Here's the drawing with two shaded views (mm, measured from the low corner). I have some questions. A direction names the side the tool comes from. Give positions to 0.01 mm unless a question says otherwise; leave off trailing zeros. Write each loop counter-clockwise with the first axis right and the second up, starting at its lowest first coordinate (ties: lowest second). Pieces come first, ordered by that corner, then holes. Notation, with made-up numbers: (15, -11.75) - (74, -11.75) arc R21 ccw to (74, 11.25) - close; hole circle Ø9 at (37, -39.5). An arc over 180 degrees is marked (long way). Answer as a JSON object with one key per item and string values. Group by question number.
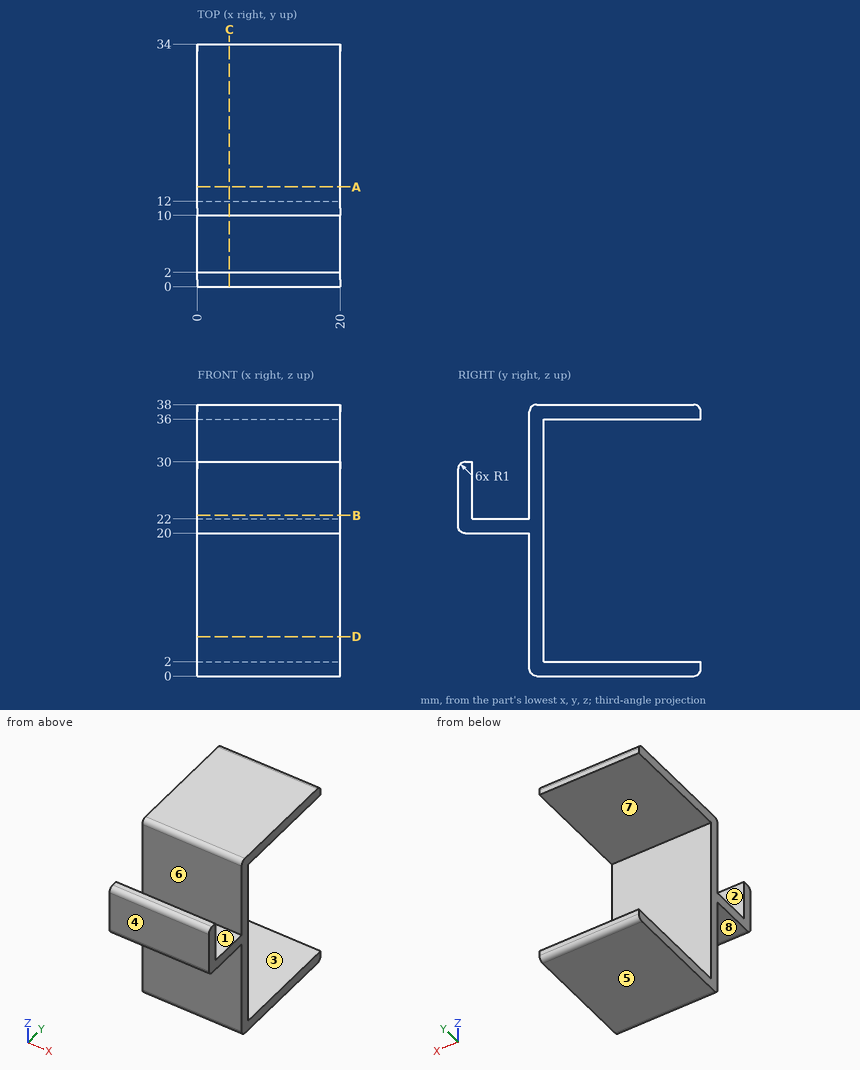
(1) I want a section at D-D, the plane z = 5.5. Please give me the cut outline in (x, y), and give its area (3 significant figures).
(2) I need wall thicknesses on L1, parallel to Z at x = 5, y = 25; L2, parallel to Y at x = 14.25, z = 3; L3, parallel to Y at x = 3.75, z = 27. Which ranges of each line are inside material? Lowest first, please.
(3) Will these pins go through, and if not, where does the flat tip stop? P1, Ø2, axis at x = 14.5, z = 15.5, coming from the -Y side; P2, Ø4, axis at x = 4, z = 29, coming from the +Y side; P3, Ø0.8, axis at x = 10.5, y = 1.5, coming from the +Z side.
(4) I want a section at B-B, the plane z = 22.5. Please give me the cut outline in (x, y).
(5) I want a section at C-C, the plane x = 4.5. Please give me the cut outline in (y, z), and give its area (3 significant figures).
(6) If we mould it in two halves opening along Y, with no side actions, what happens to the marked faces 1, 2, 3 and 4? For each: +Y half, -Y half, draft (parallel to the pull), parting line (faces both ways), or undercut.
(7) For the marked faces 5, 6, 7 and 8, which set-ups out of +Z, -Z, +X, -X, +Y, -Y let a thin tool reach every point of the face, with its end or its side?
(8) I want a section at A-A, the plane y = 14. Please give me the cut outline in (x, z).
Entries:
{
 "1": {"outline": "(0, 10) - (20, 10) - (20, 12) - (0, 12) - close", "area": "40.0 mm^2"},
 "2": {"L1": "0 to 2, 36 to 38", "L2": "10 to 12", "L3": "0 to 2, 10 to 12"},
 "3": {"P1": "y = 10", "P2": "y = 12", "P3": "z = 30"},
 "4": {"outline": "(0, 0) - (20, 0) - (20, 2) - (0, 2) - close; (0, 10) - (20, 10) - (20, 12) - (0, 12) - close"},
 "5": {"outline": "(0, 21) arc R1 ccw to (1, 20) - (10, 20) - (10, 1) arc R1 ccw to (11, 0) - (33, 0) arc R1 ccw to (34, 1) - (34, 2) - (12, 2) - (12, 36) - (34, 36) - (34, 37) arc R1 ccw to (33, 38) - (11, 38) arc R1 ccw to (10, 37) - (10, 22) - (2, 22) - (2, 30) - (1, 30) arc R1 ccw to (0, 29) - close", "area": "199 mm^2"},
 "6": {"face 1": "undercut", "face 2": "undercut", "face 3": "draft", "face 4": "-Y half"},
 "7": {"face 5": "-Z, +X, -X, +Y, -Y", "face 6": "+Z, +X, -X", "face 7": "+X, -X, +Y", "face 8": "-Z, +X, -X, -Y"},
 "8": {"outline": "(0, 0) - (20, 0) - (20, 2) - (0, 2) - close; (0, 36) - (20, 36) - (20, 38) - (0, 38) - close"}
}
